Could you check a few things on this model? Use its own coordinates, in mm. Face numbers are marked on the shaded views. A direction names the side the tool comes from. Give positions to 0.01 mm unless a question says otherwise; leave off trailing zeros. Write each loop counter-clockwise with the first axis right and the second up, starting at its lowest first coordinate (ties: lowest second). Pieces come first, ordered by that corner, then holes. Notation, with made-up numbers: (37, 68) - (43, 68) arc R20 ccw to (43, 85) - close; hole circle Ø11 at (6, 49.25). An arc over 180 degrees is marked (long way). Answer as CSV lines item,"result". Start each with the question number.
Q1. Will these pins go through, and if not, where does the flat tip stop? pin 1 Ø2 at (y, z) = (-7, -4) entering from -X; pin 2 Ø5 at (x, z) = (-45, 5) entering from +Y; pin 3 Ø5 at (x, z) = (5, -5) entering from -Y; pin 4 Ø2 at (x, z) = (4, -4.5) entering from +Y.
Q2. On a 3-axis mill with a long thin cutter (end or side, diameter ignored), from which of +Z, -Z, +X, -X, +Y, -Y can I reach the whole of each face in a straight line? I mean the marked faces 1, 2, 3 and 4. Say none if no direction works.
Q3. Imagine slicing it at D-D on y = 3. List the corners of the cut face in (x, z) for me.
Q4. If I drill on line 1 along Z through (x, y) = (5, -1); line 2 along Y through (x, z) = (-42.5, -2.75); line 3 along X through (y, z) = (10, 6.5), over which ranges is the centre line in solid material (lowest first)?
Q5. Imagine slicing it at B-B on z = -5. List the corners of the cut face in (x, y) for me, and give its area (3 significant figures).
Q6. Imagine slicing it at A-A on x = -45. List the corners of the cut face in (y, z) for me.
Q7. Imagine slicing it at C-C on x = -28.5. List the corners of the cut face in (y, z) for me, and give its area (3 significant figures).
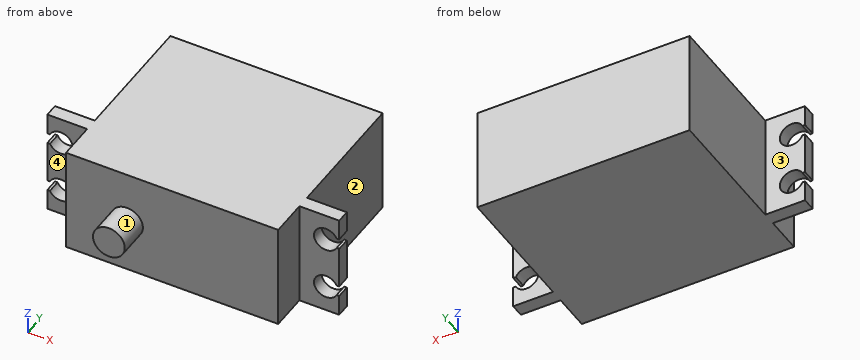
```python
from build123d import *

# Parameters (mm, degrees)
SKETCH1_W                = 40
SKETCH1_H                = 20
BOSS_EXTRUDE1_DEPTH      = 25
BOSS_EXTRUDE1_DEPTH_BACK = 9.5
BOSS_EXTRUDE2_DEPTH      = 2.5
SKETCH3_R                = 3
BOSS_EXTRUDE3_DEPTH      = 6


with BuildPart() as part:
    # Sketch1 → Boss-Extrude1 (new body, two sides)
    with BuildSketch(Plane(origin=(0, 0, 0), x_dir=(1, 0, 0), z_dir=(0, 1, 0))) as boss_extrude1_sk:
        with Locations((-20, 0)):
            Rectangle(SKETCH1_W, SKETCH1_H)
    extrude(amount=BOSS_EXTRUDE1_DEPTH)
    extrude(boss_extrude1_sk.sketch, amount=-BOSS_EXTRUDE1_DEPTH_BACK)

    # Sketch2 → Boss-Extrude2 (add)
    with BuildSketch(Plane(origin=(0, 0, 0), x_dir=(1, 0, 0), z_dir=(0, 1, 0))):
        with BuildLine():
            Line((-40, 10), (-47.5, 10))
            Line((-47.5, 10), (-47.5, 6))
            Line((-47.5, 6), (-47.015564437, 6))
            ThreePointArc((-47.015564437, 6), (-42.75, 5), (-47.015564437, 4))
            Line((-47.015564437, 4), (-47.5, 4))
            Line((-47.5, 4), (-47.5, -4))
            Line((-47.5, -4), (-47.015564437, -4))
            ThreePointArc((-47.015564437, -4), (-42.75, -5), (-47.015564437, -6))
            Line((-47.015564437, -6), (-47.5, -6))
            Line((-47.5, -6), (-47.5, -10))
            Line((-47.5, -10), (-40, -10))
            Line((-40, -10), (-40, 10))
        make_face()
        with BuildLine():
            Line((7.5, -4), (7.5, 4))
            Line((7.5, 4), (7.015564437, 4))
            ThreePointArc((7.015564437, 4), (2.75, 5), (7.015564437, 6))
            Line((7.015564437, 6), (7.5, 6))
            Line((7.5, 6), (7.5, 10))
            Line((7.5, 10), (0, 10))
            Line((0, 10), (0, -10))
            Line((0, -10), (7.5, -10))
            Line((7.5, -10), (7.5, -6))
            Line((7.5, -6), (7.015564437, -6))
            ThreePointArc((7.015564437, -6), (2.75, -5), (7.015564437, -4))
            Line((7.015564437, -4), (7.5, -4))
        make_face()
    extrude(amount=-BOSS_EXTRUDE2_DEPTH)

    # Sketch3 → Boss-Extrude3 (add)
    with BuildSketch(Plane(origin=(0, -9.5, 0), x_dir=(-1, 0, 0), z_dir=(0, -1, 0))):
        with Locations((28.5, 0)):
            Circle(SKETCH3_R)
    extrude(amount=BOSS_EXTRUDE3_DEPTH)


solid = part.part
```
Conclusion:
1,pin 1,"x = -40"
1,pin 2,"y = 0"
1,pin 3,"y = -2.5"
1,pin 4,"through"
2,face 1,"-Y"
2,face 2,"+Z, -Z, +X, +Y"
2,face 3,"+Z, -Z, -X, +Y"
2,face 4,"+Z, -Z, -X, -Y"
3,outline,"(-40, -10) - (0, -10) - (0, 10) - (-40, 10) - close"
4,line 1,"-10 to -7.25, -2.75 to 2.75, 7.25 to 10"
4,line 2,"-2.5 to 0"
4,line 3,"-40 to 0"
5,outline,"(-42.75, -2.5) - (-40, -2.5) - (-40, -9.5) - (0, -9.5) - (0, -2.5) - (2.75, -2.5) - (2.75, 0) - (0, 0) - (0, 25) - (-40, 25) - (-40, 0) - (-42.75, 0) - close"
5,area,"1,390 mm^2"
6,outline,"(-2.5, -10) - (0, -10) - (0, -7.25) - (-2.5, -7.25) - close; (-2.5, -2.75) - (0, -2.75) - (0, 2.75) - (-2.5, 2.75) - close; (-2.5, 7.25) - (0, 7.25) - (0, 10) - (-2.5, 10) - close"
7,outline,"(-15.5, -3) - (-9.5, -3) - (-9.5, -10) - (25, -10) - (25, 10) - (-9.5, 10) - (-9.5, 3) - (-15.5, 3) - close"
7,area,"726 mm^2"
